```python
from build123d import *
from OCP.BRepAlgoAPI import BRepAlgoAPI_Cut
from OCP.TopTools import TopTools_ListOfShape

# Parameters (mm, degrees)
SKETCH_283_W           = 8.41374588
SKETCH_283_H           = 7.619999886
EXTRUDE_5712_DEPTH     = 9.9695
SKETCH_4_W             = 9.683748245
SKETCH_4_H             = 5.588000536
SKETCH_4_W_2           = 9.683750153
SKETCH_4_W_3           = 1.905002594
SKETCH_4_H_2           = 7.619999886
SKETCH_4_W_4           = 43.656253815
CUT_EXTRUDE_5770_DEPTH = 8.6995
CUT_EXTRUDE_9_DEPTH    = 63.593257627
EXTRUDE_10_REACH       = 64.593
CUT_EXTRUDE_11_REACH   = 64.593
SKETCH_7_R             = 1.130300066
SKETCH_5_R             = 1.13029956
SKETCH_5_R_2           = 1.130299504
CUT_EXTRUDE_12_DEPTH   = 63.593257627


with BuildPart() as part:
    # Sketch 283 → Extrude 5712 (new body)
    with BuildSketch(Plane(origin=(0, 0, 0), x_dir=(1, 0, 0), z_dir=(0, 1, 0))):
        Polygon((43.656253815, 0), (0, 0), (0, -27.686000824), (43.656253815, -27.686000824), (43.656253815, -19.557998657), (55.245002747, -19.557998657), (55.245002747, -8.128000259), (43.656253815, -8.128000259), align=None)
        with Locations((47.863126755, -13.842999935)):
            Rectangle(SKETCH_283_W, SKETCH_283_H, mode=Mode.SUBTRACT)
    extrude(amount=EXTRUDE_5712_DEPTH)


with BuildPart() as cut_extrude_5770_tool:
    # 草图4 → Cut-Extrude 5770 (new body)
    with BuildSketch(Plane(origin=(0, 9.969499588, 0), x_dir=(1, 0, 0), z_dir=(0, 1, 0))):
        with Locations((13.73187542, -5.333999991)):
            Rectangle(SKETCH_4_W, SKETCH_4_H)
        with Locations((25.320626258, -5.333999991)):
            Rectangle(SKETCH_4_W, SKETCH_4_H)
        with Locations((36.909376145, -5.333999991)):
            Rectangle(SKETCH_4_W_2, SKETCH_4_H)
        with Locations((53.022500992, -13.842999935)):
            Rectangle(SKETCH_4_W_3, SKETCH_4_H_2)
        with Locations((21.828126907, -13.842999935)):
            Rectangle(SKETCH_4_W_4, SKETCH_4_H_2)
        with BuildLine():
            ThreePointArc((18.220330198, -23.168134689), (17.956836473, -21.282857597), (18.762168884, -19.557998657))
            Line((18.762168884, -19.557998657), (8.890001297, -19.557998657))
            Line((8.890001297, -19.557998657), (8.890001297, -23.168134689))
            Line((8.890001297, -23.168134689), (18.220330198, -23.168134689))
        make_face()
        with BuildLine():
            ThreePointArc((20.002500534, -24.883461506), (18.947446601, -24.196156461), (18.220330198, -23.168134689))
            Line((18.220330198, -23.168134689), (8.890001297, -23.168134689))
            Line((8.890001297, -23.168134689), (8.890001297, -25.145999908))
            Line((8.890001297, -25.145999908), (20.002500534, -25.145999908))
            Line((20.002500534, -25.145999908), (20.002500534, -24.883461506))
        make_face()
        with BuildLine():
            ThreePointArc((30.927521198, -23.168134689), (30.663518149, -21.282433428), (31.470916179, -19.557998657))
            Line((31.470916179, -19.557998657), (23.782831176, -19.557998657))
            ThreePointArc((23.782831176, -19.557998657), (24.407616627, -20.592090361), (24.625300686, -21.78049945))
            ThreePointArc((24.625300686, -21.78049945), (24.549281168, -22.490413257), (24.324669862, -23.168134689))
            Line((24.324669862, -23.168134689), (30.927521198, -23.168134689))
        make_face()
        with BuildLine():
            ThreePointArc((32.772350311, -24.904129054), (31.679314783, -24.217449589), (30.927521198, -23.168134689))
            Line((30.927521198, -23.168134689), (24.324669862, -23.168134689))
            ThreePointArc((24.324669862, -23.168134689), (23.597554208, -24.19615574), (22.54250145, -24.883460719))
            Line((22.54250145, -24.883460719), (22.54250145, -25.145999908))
            Line((22.54250145, -25.145999908), (32.772350311, -25.145999908))
            Line((32.772350311, -25.145999908), (32.772350311, -24.904129054))
        make_face()
        with BuildLine():
            Line((41.751251221, -25.145999908), (41.751251221, -23.168134689))
            Line((41.751251221, -23.168134689), (37.017476717, -23.168134689))
            ThreePointArc((37.017476717, -23.168134689), (36.671360521, -23.758773077), (36.212287817, -24.266613976))
            Line((36.212287817, -24.266613976), (36.221363068, -24.267242432))
            Line((36.221363068, -24.267242432), (36.150205492, -24.321171358))
            ThreePointArc((36.150205492, -24.321171358), (35.993676848, -24.447381385), (35.8298504, -24.563962181))
            Line((35.8298504, -24.563962181), (35.758705139, -24.617881775))
            Line((35.758705139, -24.617881775), (35.749340746, -24.616033322))
            ThreePointArc((35.749340746, -24.616033322), (35.501472205, -24.757017499), (35.242500305, -24.876386285))
            Line((35.242500305, -24.876386285), (35.242500305, -25.145999908))
            Line((35.242500305, -25.145999908), (41.751251221, -25.145999908))
        make_face()
        with BuildLine():
            Line((41.751251221, -23.168134689), (41.751251221, -19.557998657))
            Line((41.751251221, -19.557998657), (36.474081737, -19.557998657))
            ThreePointArc((36.474081737, -19.557998657), (37.10046612, -20.591699149), (37.318754037, -21.780498749))
            ThreePointArc((37.318754037, -21.780498749), (37.242567409, -22.490481412), (37.017476717, -23.168134689))
            Line((37.017476717, -23.168134689), (41.751251221, -23.168134689))
        make_face()
    extrude(amount=-CUT_EXTRUDE_5770_DEPTH)


with BuildPart() as part_1:
    add(part.part)

    # Cut-Extrude 5770: cut by cut_extrude_5770_tool, with a tolerance
    cut_extrude_5770_stock = TopTools_ListOfShape()
    cut_extrude_5770_stock.Append(part_1.part.wrapped)
    cut_extrude_5770_tools = TopTools_ListOfShape()
    cut_extrude_5770_tools.Append(cut_extrude_5770_tool.part.wrapped)
    cut_extrude_5770_cut = BRepAlgoAPI_Cut()
    cut_extrude_5770_cut.SetArguments(cut_extrude_5770_stock)
    cut_extrude_5770_cut.SetTools(cut_extrude_5770_tools)
    cut_extrude_5770_cut.SetFuzzyValue(0.00001)
    cut_extrude_5770_cut.Build()
    add(Compound.cast(cut_extrude_5770_cut.Shape()).solids(), mode=Mode.REPLACE)

    # Sketch 3431 → 拉伸9 (cut, through all)
    with BuildSketch(Plane(origin=(0, 0, 0), x_dir=(0, 0, -1), z_dir=(1, 0, 0))):
        Polygon((0, 0), (-3.628601313, 0), (0, 9.969499588), align=None)
    cut_extrude_9 = extrude(amount=CUT_EXTRUDE_9_DEPTH, mode=Mode.SUBTRACT)

    # 拉伸10: up to this face of the body (flat: up to its plane)
    extrude_10_end = Plane(part_1.part.faces().sort_by_distance((43.656253815, 5.462221292, 4.884257746))[0])
    # 右视标记<6> → 拉伸10 (add, up to the picked face)
    with BuildSketch(Plane(origin=(0, 0, 0), x_dir=(0, 0, -1), z_dir=(1, 0, 0)), mode=Mode.PRIVATE) as extrude_10_sk1:
        Polygon((-8.128000259, 1.269999862), (-8.128000259, 0), (-3.628601313, 0), (0, 9.969499588), (-2.539999723, 9.969499588), (-2.539999723, 6.704138756), (-4.517864227, 1.269999862), align=None)
    extrude_10_tool1 = split(extrude(extrude_10_sk1.sketch, amount=EXTRUDE_10_REACH, mode=Mode.PRIVATE), bisect_by=extrude_10_end, keep=Keep.BOTH, mode=Mode.PRIVATE)
    extrude_10 = extrude_10_tool1.solids().sort_by(Axis((0, 4.424317, 3.31525), (1, 0, 0)))[0]
    add(extrude_10)

    # 右视标记<7> → 拉伸11 (cut, up to next)
    with BuildSketch(Plane(origin=(0, 0, 0), x_dir=(0, 0, -1), z_dir=(1, 0, 0)), mode=Mode.PRIVATE) as cut_extrude_11_sk1:
        with Locations(Location((-5.905499899, 5.258642622, 0), (0, 0, 180))):
            Circle(SKETCH_7_R)
    cut_extrude_11_tool1 = extrude(cut_extrude_11_sk1.sketch, amount=CUT_EXTRUDE_11_REACH, mode=Mode.PRIVATE) & part_1.part
    cut_extrude_11 = cut_extrude_11_tool1.solids().sort_by_distance((0, 5.258643, 5.9055))[0]
    add(cut_extrude_11, mode=Mode.SUBTRACT)

    # 镜向2: 拉伸9, 拉伸10, 拉伸11 across plane
    add(cut_extrude_9.mirror(Plane.XY.offset(13.843000412)), mode=Mode.SUBTRACT)
    add(extrude_10.mirror(Plane.XY.offset(13.843000412)))
    add(cut_extrude_11.mirror(Plane.XY.offset(13.843000412)), mode=Mode.SUBTRACT)

    # 上视标记<5> → 拉伸12 (cut, through all)
    with BuildSketch(Plane(origin=(0, 0, 0), x_dir=(1, 0, 0), z_dir=(0, 1, 0))):
        with Locations(Location((21.27250003, -21.78049945, 0), (0, 0, 270))):
            Circle(SKETCH_5_R)
        with Locations(Location((33.972498958, -21.780498749, 0), (0, 0, 270))):
            Circle(SKETCH_5_R_2)
    extrude(amount=CUT_EXTRUDE_12_DEPTH, mode=Mode.SUBTRACT)


solid = part_1.part
```
Input: part model. Units: mm. Frame: model coordinates. A direction names the side the tool comes from. Give positions to 0.01 mm unless a question says otherwise; leave off trailing zeros. Order: outer loops, then holes, each group sorted by start corner. A loop starts at its lowest first (then second) coordinate and runs counter-clockwise, first axis right, second up. Notation, with made-up numbers: (32, 45.5) - (81, 45.5) arc R21 ccw to (81, 56.5) - close; hole circle Ø3 at (-39, 85). An arc over 180 degrees is marked (long way). One line per item, written item: value.
1. Reachability of faces 1 (the face through (43.656, 1, 14)), 2 (the face through (22, 1.27, 14)), 3 (the face through (18.574, 6, 5)) from +Z, -Z, +X, -X, +Y, -Y: full face, straight path, thin tool, end or side. Return the list, or none.
Determined:
face 1: +Y, -Y
face 2: -X, +Y
face 3: +Y
2. Cut plane C-C, the plane y = 2.75. Give the number of separate pieces and of enclosed holes in the cut face, and give its area (3 significant figures).
Determined:
separate pieces: 1
enclosed holes: 8
area: 487 mm2
3. Line query: probe 1 along X at (y, z) = (2.25, 8); probe 2 along Z at (x, y) = (46, 5.25); probe 3 along X at (y, z) = (4.5, 5.5). Output: solid intervals per line, ascending.
Determined:
probe 1: 0 to 8.89, 18.57 to 20.48, 30.16 to 32.07, 41.75 to 43.66
probe 2: 8.13 to 10.03, 17.65 to 19.56
probe 3: 18.57 to 20.48, 30.16 to 32.07, 41.75 to 43.66
4. Draft query along Z for faces 4 (the face through (50, 5, 8.128)), 5 (the face through (55.245, 5, 14)), 6 (the face through (25, 6, 8.128)). Return one class per face: released by +Z, released by -Z, zero draft, split by the parting line, or undercut.
Determined:
face 4: released by -Z
face 5: zero draft
face 6: undercut
5. Pin query (flat end, axial travel): pin 1 Ø5 at (y, z) = (5, 3) entering from +X; pin 2 Ø3 at (x, y) = (31, 4.5) entering from -Z; pin 3 Ø2.5 at (x, y) = (25.5, 4) entering from +Z. Return the tip coordinate at first contact, or that it passes through.
Determined:
pin 1: x = 43.66
pin 2: z = 1.44
pin 3: z = 25.97
6. Cut plane B-B, the plane x = 25.5. Output: boundary loops of the cut face in (y, z), and give its area (3 significant figures).
Determined:
outline: (0, 3.63) - (9.97, 0) - (9.97, 2.54) - (6.7, 2.54) - (1.27, 4.52) - (1.27, 8.13) - (9.97, 8.13) - (9.97, 10.03) - (1.27, 10.03) - (1.27, 17.65) - (9.97, 17.65) - (9.97, 19.56) - (1.27, 19.56) - (1.27, 23.17) - (6.7, 25.15) - (9.97, 25.15) - (9.97, 27.69) - (0, 24.06) - close
area: 87.1 mm2
7. Cut plane A-A, the plane z = 15.5. Output: boundary loops of the cut face in (x, y) (1 decimal), and give its area (3 significant figures).
Determined:
outline: (0, 0) - (43.7, 0) - (43.7, 1.3) - (0, 1.3) - close; (52.1, 0) - (55.2, 0) - (55.2, 10) - (54, 10) - (54, 1.3) - (52.1, 1.3) - close
area: 70.5 mm2
